```python
from build123d import *

# Parameters (mm, degrees)
F1_DEPTH = 50.8
F2_R     = 16.3806904911
F3_DEPTH = 10.16
F6_SIZE  = 6.35


# Not quite as in the source:
# - a fillet or chamfer that OpenCascade refuses, or shapes differently, is made with other operations: its cross-section is extruded or revolved along the edge and cut away or added


with BuildPart() as f1:
    # F0 (on Front) → F1 (new body)
    with BuildSketch(Plane.XZ):
        Polygon((12.7, -7.3323484187), (12.7, 7.3323484187), (0, 14.6646968374), (-12.7, 7.3323484187), (-12.7, -7.3323484187), (0, -14.6646968374), align=None)
    extrude(amount=F1_DEPTH)

    # F2 (on Front) + F1_face (on face) + F1_face1 (on face) → F3 (join)
    with BuildSketch(Plane.XZ):
        Circle(F2_R)
    with BuildSketch(Plane(origin=(0, 0, 0), x_dir=(1, 0, 0), z_dir=(0, 1, 0))):
        Polygon((12.7, -7.3323484187), (12.7, 7.3323484187), (0, 14.6646968374), (-12.7, 7.3323484187), (-12.7, -7.3323484187), (0, -14.6646968374), align=None)
    with BuildSketch(Plane.XZ.offset(50.8)):
        Polygon((12.7, -7.3323484187), (12.7, 7.3323484187), (0, 14.6646968374), (-12.7, 7.3323484187), (-12.7, -7.3323484187), (0, -14.6646968374), align=None)
    extrude(amount=-F3_DEPTH, dir=(0, -1, 0))

    # F4: fillet of radius 2.54 on 3 edges, made by hand

    # F4_s1 → F4_t2 (revolve, cut)
    with BuildSketch(Plane.XY):
        with BuildLine():
            ThreePointArc((16.3806904911, 7.62), (15.6367417153, 9.4160512242), (13.8406904911, 10.16))
            Line((13.8406904911, 10.16), (16.3806904911, 10.16))
            Line((16.3806904911, 10.16), (16.3806904911, 7.62))
        make_face()
    revolve(axis=Axis((0, 10.16, 0), (0, -1, 0)), mode=Mode.SUBTRACT)


with BuildPart() as f4_tool4:
    # F4_s5 → F4_t6 (revolve)
    with BuildSketch(Plane.XY):
        with BuildLine():
            ThreePointArc((13.8406904911, 0), (15.6367417153, 0.7439487758), (16.3806904911, 2.54))
            Line((16.3806904911, 2.54), (16.3806904911, 0))
            Line((16.3806904911, 0), (13.8406904911, 0))
        make_face()
    revolve(axis=Axis((0, 0, 0), (0, -1, 0)))

    split(bisect_by=Plane.YZ.offset(12.7), keep=Keep.TOP)


with BuildPart() as f1_1:
    add(f1.part)

    # F4_t3: cut F4_tool4
    add(f4_tool4.part, mode=Mode.SUBTRACT)


with BuildPart() as f4_tool9:
    # F4_s10 → F4_t11 (revolve)
    with BuildSketch(Plane.XY):
        with BuildLine():
            ThreePointArc((13.8406904911, 0), (15.6367417153, 0.7439487758), (16.3806904911, 2.54))
            Line((16.3806904911, 2.54), (16.3806904911, 0))
            Line((16.3806904911, 0), (13.8406904911, 0))
        make_face()
    revolve(axis=Axis((0, 0, 0), (0, -1, 0)))

    split(bisect_by=Plane(origin=(6.35, 0, 10.9985226281), x_dir=(0, 1, 0), z_dir=(0.5, 0, 0.8660254038)), keep=Keep.TOP)


with BuildPart() as f1_2:
    add(f1_1.part)

    # F4_t8: cut F4_tool9
    add(f4_tool9.part, mode=Mode.SUBTRACT)


with BuildPart() as f4_tool14:
    # F4_s15 → F4_t16 (revolve)
    with BuildSketch(Plane.XY):
        with BuildLine():
            ThreePointArc((13.8406904911, 0), (15.6367417153, 0.7439487758), (16.3806904911, 2.54))
            Line((16.3806904911, 2.54), (16.3806904911, 0))
            Line((16.3806904911, 0), (13.8406904911, 0))
        make_face()
    revolve(axis=Axis((0, 0, 0), (0, -1, 0)))

    split(bisect_by=Plane(origin=(6.35, 0, -10.9985226281), x_dir=(0, 1, 0), z_dir=(0.5, 0, -0.8660254038)), keep=Keep.TOP)


with BuildPart() as f1_3:
    add(f1_2.part)

    # F4_t13: cut F4_tool14
    add(f4_tool14.part, mode=Mode.SUBTRACT)


with BuildPart() as f4_tool19:
    # F4_s20 → F4_t21 (revolve)
    with BuildSketch(Plane.XY):
        with BuildLine():
            ThreePointArc((13.8406904911, 0), (15.6367417153, 0.7439487758), (16.3806904911, 2.54))
            Line((16.3806904911, 2.54), (16.3806904911, 0))
            Line((16.3806904911, 0), (13.8406904911, 0))
        make_face()
    revolve(axis=Axis((0, 0, 0), (0, -1, 0)))

    split(bisect_by=Plane(origin=(-6.35, 0, 10.9985226281), x_dir=(0, 1, 0), z_dir=(-0.5, 0, 0.8660254038)), keep=Keep.TOP)


with BuildPart() as f1_4:
    add(f1_3.part)

    # F4_t18: cut F4_tool19
    add(f4_tool19.part, mode=Mode.SUBTRACT)


with BuildPart() as f4_tool24:
    # F4_s25 → F4_t26 (revolve)
    with BuildSketch(Plane.XY):
        with BuildLine():
            ThreePointArc((13.8406904911, 0), (15.6367417153, 0.7439487758), (16.3806904911, 2.54))
            Line((16.3806904911, 2.54), (16.3806904911, 0))
            Line((16.3806904911, 0), (13.8406904911, 0))
        make_face()
    revolve(axis=Axis((0, 0, 0), (0, -1, 0)))

    split(bisect_by=Plane(origin=(-6.35, 0, -10.9985226281), x_dir=(0, 1, 0), z_dir=(-0.5, 0, -0.8660254038)), keep=Keep.TOP)


with BuildPart() as f1_5:
    add(f1_4.part)

    # F4_t23: cut F4_tool24
    add(f4_tool24.part, mode=Mode.SUBTRACT)


with BuildPart() as f4_tool29:
    # F4_s30 → F4_t31 (revolve)
    with BuildSketch(Plane.XY):
        with BuildLine():
            ThreePointArc((13.8406904911, 0), (15.6367417153, 0.7439487758), (16.3806904911, 2.54))
            Line((16.3806904911, 2.54), (16.3806904911, 0))
            Line((16.3806904911, 0), (13.8406904911, 0))
        make_face()
    revolve(axis=Axis((0, 0, 0), (0, -1, 0)))

    split(bisect_by=Plane.YZ.offset(-12.7), keep=Keep.BOTTOM)


with BuildPart() as f1_6:
    add(f1_5.part)

    # F4_t28: cut F4_tool29
    add(f4_tool29.part, mode=Mode.SUBTRACT)

    # F6
    f6_edges = [f1_6.edges().sort_by_distance(p)[0] for p in [
        (12.7, -50.8, 0),
        (6.35, -50.8, 10.998523),
        (-6.35, -50.8, 10.998523),
        (-12.7, -50.8, 0),
        (-6.35, -50.8, -10.998523),
        (6.35, -50.8, -10.998523),
    ]]
    chamfer(f6_edges, length=F6_SIZE)


solid = f1_6.part
```
The model under review builds one solid part; all positions refer to its coordinate system, in mm. A direction names the side the tool comes from. Round coordinates to 2 decimals unless told otherwise and drop trailing zeros. Loops run counter-clockwise (first coordinate to the right, second up) from the corner with the lowest first, then second, coordinate; pieces in that order, holes last.
1) Clearance check with flat-ended pins moving along their axes: P1, Ø0.9, axis at x = -13, z = -1, coming from the -Y side; P2, Ø10, axis at y = -3.5, z = 5.5, coming from the -X side; P3, Ø6, axis at x = -3.5, z = 9.5, coming from the -Y side. State where each tip first meets the part, or that it passes through.
Values follow:
P1: stops at y = -44.6
P2: stops at x = -15.54
P3: stops at y = -50.17
2) Tool access review of faces 1 (the face through (10.19, -46.96, -0.1)), 2 (the face through (7, 0, -11)), 3 (the face through (7, 0, 11)), 4 (the face through (-7, 0, 11)), 5 (the face through (-7, 0, -11)): name each direction out of +Z, -Z, +X, -X, +Y, -Y from which nothing blocks a thin tool from reaching the whole face with its end or side.
Values follow:
face 1: +Z, -Z, +X, -Y
face 2: -Z, +X, -Y
face 3: +Z, +X, -Y
face 4: +Z, -X, -Y
face 5: -Z, -X, -Y
3) Consider section B-B on y = -2. State the section outline as (x, z) points.
Values follow:
outline: (-12.7, -7.33) - (0, -14.66) - (12.7, -7.33) - (12.7, 7.33) - (0, 14.66) - (-12.7, 7.33) - close
4) Consider section A-A on z = 0. State the section outline as (x, y) points, then the cut area to 3 significant figures.
Values follow:
outline: (-16.38, 2.54) arc R2.54 ccw to (-13.84, 0) - (-12.7, 0) - (-12.7, -44.45) - (-6.35, -50.8) - (6.35, -50.8) - (12.7, -44.45) - (12.7, 0) - (13.84, 0) arc R2.54 ccw to (16.38, 2.54) - (16.38, 7.62) arc R2.54 ccw to (13.84, 10.16) - (-13.84, 10.16) arc R2.54 ccw to (-16.38, 7.62) - close
area: 1,580 mm2
5) Wall thickness on line 1 along X through (y, z) = (-9, -7); line 2 along Y through (x, z) = (4, 13); line 3 along X through (y, z) = (-43.5, 11): over which ranges is each line inside the solid? List them lowest first.
Values follow:
line 1: x = -12.7 to 12.7
line 2: y = 0 to 10.16
line 3: x = -6.35 to 6.35
